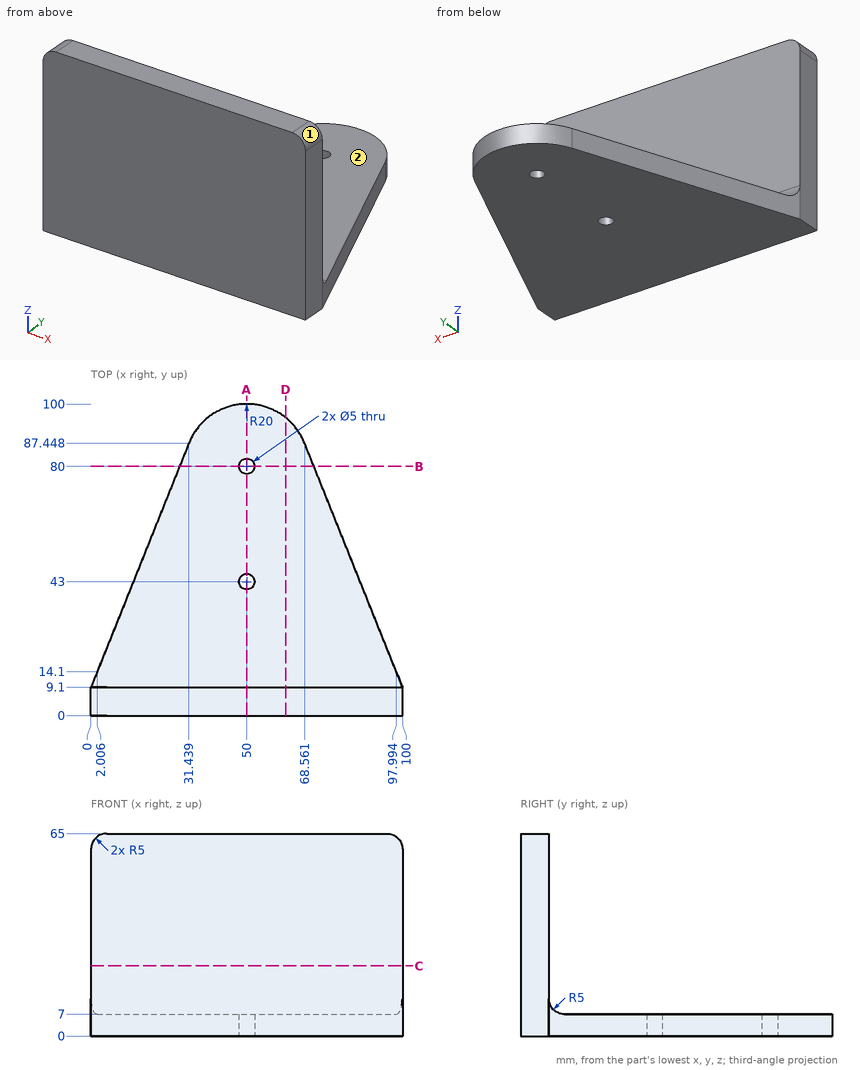
Here's the drawing with two shaded views (mm, measured from the low corner). I have some questions. A direction names the side the tool comes from. Coordinates: 2 decimals unless noted, no trailing zeros. Write each loop counter-clockwise with the first axis right and the second up, starting at its lowest first coordinate (ties: lowest second). Pieces come first, ordered by that corner, then holes. Notation, with made-up numbers: (80.5, 82.5) -> (138.5, 82.5) arc R32 ccw to (138.5, 120.5) -> close; hole circle Ø7 at (39, 35.5). An arc over 180 degrees is marked (long way). Use a Markdown table: item, result. Add a question column.
(1) If we section it at B-B, the plane y = 80: Write out the boundary of the cut face in (x, z).
(2) For the marked faces 1 and 2, which set-ups out of +Z, -Z, +X, -X, +Y, -Y let a thin tool reach every point of the face, with its end or its side?
(3) If we section it at D-D, the plane x = 62.5: Write out the boundary of the cut face in (y, z).
(4) Please list where these lines run through material, in increasing order: line 1 (Y direction, x = 50, z = 5); line 2 (Y direction, x = 78, z = 31); line 3 (Z direction, x = 29.5, y = 73).
(5) If we section it at A-A, the plane x = 50: Write out the boundary of the cut face in (y, z).
(6) If we section it at C-C, the plane z = 22.5: Write out the boundary of the cut face in (x, y).
(7) I'm going to push flat-ended pins straight in: P1, Ø8, axis at y = 82.5, z = 8.5, coming from the -X side (1 decimal); P2, Ø6, axis at x = 50, y = 80, coming from the +Z side. Where does each tip first touch, or does it pass through?
Outcome:
| question | item | result |
|---|---|---|
| 1 | outline | (28.45, 0) -> (47.5, 0) -> (47.5, 7) -> (28.45, 7) -> close; (52.5, 0) -> (71.55, 0) -> (71.55, 7) -> (52.5, 7) -> close |
| 2 | face 1 | +Z, +X, +Y, -Y |
| 2 | face 2 | +Z, +X, -X, +Y |
| 3 | outline | (0, 0) -> (95.61, 0) -> (95.61, 7) -> (14.1, 7) arc R5 cw to (9.1, 12) -> (9.1, 65) -> (0, 65) -> close |
| 4 | line 1 | y = 0 to 40.5, 45.5 to 77.5, 82.5 to 100 |
| 4 | line 2 | y = 0 to 9.1 |
| 4 | line 3 | z = 0 to 7 |
| 5 | outline | (0, 0) -> (40.5, 0) -> (40.5, 7) -> (14.1, 7) arc R5 cw to (9.1, 12) -> (9.1, 65) -> (0, 65) -> close; (45.5, 0) -> (77.5, 0) -> (77.5, 7) -> (45.5, 7) -> close; (82.5, 0) -> (100, 0) -> (100, 7) -> (82.5, 7) -> close |
| 6 | outline | (0, 0) -> (100, 0) -> (100, 9.1) -> (0, 9.1) -> close |
| 7 | P1 | stops at x = 28 |
| 7 | P2 | stops at z = 7 |
